Source: CAD feature listing. Evaluate the final solid. Frame: model axes, mm. A direction names the side the tool comes from. Coordinates: 2 decimals unless noted, no trailing zeros. Order: outer loops, then holes, each group sorted by start corner. A loop starts at its lowest first (then second) coordinate and runs counter-clockwise, first axis right, second up. Notation, with made-up numbers: (14, -36) -> (59, -36) arc R32 ccw to (59, -10) -> close; hole circle Ø9 at (5, -7.75). An arc over 180 degrees is marked (long way). Write item = value, one per line. Start each with the question number.
Item 1: Section query C-C (y = 59). Output: boundary loops of the cut face in (x, z).
Item 2: Section query A-A (z = -15). Output: boundary loops of the cut face in (x, y), then the cut area to 3 significant figures.
Item 3: Section query D-D (x = -73). Output: boundary loops of the cut face in (y, z).
Item 4: Contact query for flat-ended pins moving along their axis: pin 1 (3.5 mm diameter, centred on y = -77, z = -1.5, fed in from -X); pin 2 (1 mm diameter, centred on x = -54, y = -45.5, fed in from -Z); pin 3 (2.5 mm diameter, centred on y = -84.5, z = -2, fed in from +X). Output: stop coordinate, or through.
Item 5: Mould query, pull axis Z, two halves, no side actions, for faces 1 (the flat face through (1, -1, -3)), 2 (the flat face through (-1, -1, 0)), 3 (the cylindrical face through (-96.98, -83.04, -14.41)). Classes: released by +Z, released by -Z, zero draft, split by the parting line, or undercut.
Item 6: Set-up query: faces 4 (the flat face through (-95.5, -1, -14)), 5 (the flat face through (98.5, -1, -14)). Return all of +Z, -Z, +X, -X, +Y, -Y with unobstructed straight access to the full face (end or side cutting, diameter ignored); none if empty.
Item 7: Ray query, line 1 along Y through (x, z) = (96.45, -15); line 2 along X through (y, z) = (78.5, -4.5); line 3 along Z through (x, y) = (-61, 34). Return the intervals inside material, ascending. Write a range as [from, to].
Item 8: Section query B-B (y = -87.5). Output: boundary loops of the cut face in (x, z), then the cut area to 3 significant figures.
```python
from build123d import *

# Parameters (mm, degrees)
BASE_FLANGE1_START = -103.5
BASE_FLANGE1_DEPTH = 207
CUT_EXTRUDE1_REACH = 225.934
SKETCH6_R          = 4.5
CUT_EXTRUDE2_REACH = 147.05
FILLET1_R          = 3
FILLET2_R          = 3


# Read off the part's stored shape, not the designer's step: Base-Flange1
with BuildPart() as part:
    # Base-Flange1 outline → Base-Flange1 (new body)
    with BuildSketch(Plane(origin=(0, 0, 0), x_dir=(1, 0, 0), z_dir=(0, 1, 0)).offset(BASE_FLANGE1_START)):
        with BuildLine():
            Line((-95.5, 4), (-95.5, 25))
            Line((-95.5, 25), (-98.5, 25))
            Line((-98.5, 25), (-98.5, 4))
            ThreePointArc((-98.5, 4), (-97.328427125, 1.171572875), (-94.5, 0))
            Line((-94.5, 0), (94.5, 0))
            ThreePointArc((94.5, 0), (97.328427125, 1.171572875), (98.5, 4))
            Line((98.5, 4), (98.5, 25))
            Line((98.5, 25), (95.5, 25))
            Line((95.5, 25), (95.5, 4))
            ThreePointArc((95.5, 4), (95.207106781, 3.292893219), (94.5, 3))
            Line((94.5, 3), (-94.5, 3))
            ThreePointArc((-94.5, 3), (-95.207106781, 3.292893219), (-95.5, 4))
        make_face()
    extrude(amount=BASE_FLANGE1_DEPTH)

    # Cut-Extrude1: up to this face of the body (flat: up to its plane)
    cut_extrude1_end = Plane(part.part.faces().sort_by_distance((-98.5, 0, -14.5))[0])
    # Sketch6 → Cut-Extrude1 (cut, up to the picked face)
    with BuildSketch(Plane(origin=(98.5, 0, 0), x_dir=(0, 0, -1), z_dir=(1, 0, 0)), mode=Mode.PRIVATE) as cut_extrude1_sk1:
        with Locations((15, 87.5)):
            Circle(SKETCH6_R)
    cut_extrude1_tool1 = split(extrude(cut_extrude1_sk1.sketch, amount=-CUT_EXTRUDE1_REACH, mode=Mode.PRIVATE), bisect_by=cut_extrude1_end, keep=Keep.BOTH, mode=Mode.PRIVATE)
    # Sketch6 → Cut-Extrude1 (cut, up to the picked face)
    with BuildSketch(Plane(origin=(98.5, 0, 0), x_dir=(0, 0, -1), z_dir=(1, 0, 0)), mode=Mode.PRIVATE) as cut_extrude1_sk2:
        with Locations((15, -87.5)):
            Circle(SKETCH6_R)
    cut_extrude1_tool2 = split(extrude(cut_extrude1_sk2.sketch, amount=-CUT_EXTRUDE1_REACH, mode=Mode.PRIVATE), bisect_by=cut_extrude1_end, keep=Keep.BOTH, mode=Mode.PRIVATE)
    add(cut_extrude1_tool1.solids().sort_by(Axis((98.5, 87.5, -15), (-1, 0, 0)))[0], mode=Mode.SUBTRACT)
    add(cut_extrude1_tool2.solids().sort_by(Axis((98.5, -87.5, -15), (-1, 0, 0)))[0], mode=Mode.SUBTRACT)

    # Sketch7 → Cut-Extrude2 (cut, up to next)
    with BuildSketch(Plane.XY, mode=Mode.PRIVATE) as cut_extrude2_sk1:
        with BuildLine():
            Line((24.494899552, 103.5), (24.494899552, 53.999895909))
            ThreePointArc((24.494899552, 53.999895909), (0, 29), (-24.494899552, 53.999895909))
            Line((-24.494899552, 53.999895909), (-24.494899552, 103.5))
            Line((-24.494899552, 103.5), (24.494899552, 103.5))
        make_face()
    cut_extrude2_tool1 = extrude(cut_extrude2_sk1.sketch, amount=-CUT_EXTRUDE2_REACH, mode=Mode.PRIVATE) & part.part
    # Sketch7 → Cut-Extrude2 (cut, up to next)
    with BuildSketch(Plane.XY, mode=Mode.PRIVATE) as cut_extrude2_sk2:
        with BuildLine():
            Line((24.494899552, -103.5), (24.494899552, -53.999895909))
            ThreePointArc((24.494899552, -53.999895909), (0, -29), (-24.494899552, -53.999895909))
            Line((-24.494899552, -53.999895909), (-24.494899552, -103.5))
            Line((-24.494899552, -103.5), (24.494899552, -103.5))
        make_face()
    cut_extrude2_tool2 = extrude(cut_extrude2_sk2.sketch, amount=-CUT_EXTRUDE2_REACH, mode=Mode.PRIVATE) & part.part
    add(cut_extrude2_tool1.solids().sort_by_distance((0, 68.661453, 0))[0], mode=Mode.SUBTRACT)
    add(cut_extrude2_tool2.solids().sort_by_distance((0, -68.661453, 0))[0], mode=Mode.SUBTRACT)

    # Fillet1
    fillet1_edges = [part.edges().sort_by_distance(p)[0] for p in [
        (97, -103.5, -25),
        (-97, -103.5, -25),
        (97, 103.5, -25),
        (-97, 103.5, -25),
    ]]
    fillet(fillet1_edges, radius=FILLET1_R)

    # Fillet2
    fillet2_edges = [part.edges().sort_by_distance(p)[0] for p in [
        (-24.494899552, 103.5, -1.5),
        (24.494899552, 103.5, -1.5),
        (24.494899552, -103.5, -1.5),
        (-24.494899552, -103.5, -1.5),
    ]]
    fillet(fillet2_edges, radius=FILLET2_R)


solid = part.part
```
Computed:
q1.outline = (-98.5, -25) -> (-95.5, -25) -> (-95.5, -4) arc R1 cw to (-94.5, -3) -> (-24.49, -3) -> (-24.49, 0) -> (-94.5, 0) arc R4 ccw to (-98.5, -4) -> close; (24.49, -3) -> (94.5, -3) arc R1 cw to (95.5, -4) -> (95.5, -25) -> (98.5, -25) -> (98.5, -4) arc R4 ccw to (94.5, 0) -> (24.49, 0) -> close
q2.outline = (-98.5, -103.5) -> (-95.5, -103.5) -> (-95.5, -92) -> (-98.5, -92) -> close; (-98.5, -83) -> (-95.5, -83) -> (-95.5, 83) -> (-98.5, 83) -> close; (-98.5, 92) -> (-95.5, 92) -> (-95.5, 103.5) -> (-98.5, 103.5) -> close; (95.5, -103.5) -> (98.5, -103.5) -> (98.5, -92) -> (95.5, -92) -> close; (95.5, -83) -> (98.5, -83) -> (98.5, 83) -> (95.5, 83) -> close; (95.5, 92) -> (98.5, 92) -> (98.5, 103.5) -> (95.5, 103.5) -> close
q2.area = 1,130 mm^2
q3.outline = (-103.5, -3) -> (103.5, -3) -> (103.5, 0) -> (-103.5, 0) -> close
q4.pin_1 = -98.43
q4.pin_2 = -3
q4.pin_3 = 98.43
q5.face_1 = released by -Z
q5.face_2 = released by +Z
q5.face_3 = undercut
q6.face_4 = -Z, +Y, -Y
q6.face_5 = +Z, -Z, +X, +Y, -Y
q7.line_1 = [-103.5, -92], [-83, 83], [92, 103.5]
q7.line_2 = [-98.5, -95.5], [95.5, 98.5]
q7.line_3 = [-3, 0]
q8.outline = (-98.5, -25) -> (-95.5, -25) -> (-95.5, -19.5) -> (-98.5, -19.5) -> close; (-98.5, -10.5) -> (-95.5, -10.5) -> (-95.5, -4) arc R1 cw to (-94.5, -3) -> (-24.49, -3) -> (-24.49, 0) -> (-94.5, 0) arc R4 ccw to (-98.5, -4) -> close; (24.49, -3) -> (94.5, -3) arc R1 cw to (95.5, -4) -> (95.5, -10.5) -> (98.5, -10.5) -> (98.5, -4) arc R4 ccw to (94.5, 0) -> (24.49, 0) -> close; (95.5, -25) -> (98.5, -25) -> (98.5, -19.5) -> (95.5, -19.5) -> close
q8.area = 516 mm^2
